Input: part model. Units: mm. Frame: model coordinates. A direction names the side the tool comes from. Round coordinates to 2 decimals unless told otherwise and drop trailing zeros. Order: outer loops, then holes, each group sorted by start corner. A loop starts at its lowest first (then second) coordinate and runs counter-clockwise, first axis right, second up. Notation, with made-up numbers: M -18.75,63.25 L 30.25,63.25 A28 ccw 30.25,85.25 Z; hole C 83,-18.75 d3. An arc over 180 degrees is marked long. One line per question, with ' | ' between items.
```python
from build123d import *

# Parameters (mm, degrees)
BOSS_EXTRUDE1_DEPTH = 20
SKETCH2_W           = 1
SKETCH2_H           = 2.5
SKETCH2_H_2         = 10
BOSS_EXTRUDE2_DEPTH = 2.5
SKETCH2_3_R         = 2.5
CUT_EXTRUDE1_DEPTH  = 35.641016151
SKETCH3_W           = 1
SKETCH3_H           = 10
BOSS_EXTRUDE3_DEPTH = 2.5
SKETCH4_W           = 1
SKETCH4_H           = 10
SKETCH4_W_2         = 10
SKETCH4_H_2         = 1
BOSS_EXTRUDE4_DEPTH = 2.5
SKETCH4_3_R         = 2.5
CUT_EXTRUDE2_DEPTH  = 37.142080737
SKETCH5_R           = 6
CUT_EXTRUDE3_DEPTH  = 17
SKETCH6_R           = 6
CUT_EXTRUDE4_DEPTH  = 17
SKETCH7_R           = 6
CUT_EXTRUDE5_DEPTH  = 17


with BuildPart() as part:
    # Sketch1 → Boss-Extrude1 (new body)
    with BuildSketch(Plane(origin=(0, 0, 0), x_dir=(1, 0, 0), z_dir=(0, 1, 0))):
        Polygon((0, 7.5), (3, 7.5), (3, 12.5), (0, 12.5), (0, 20), (20, 20), (20, 0), (0, 0), align=None)
    extrude(amount=BOSS_EXTRUDE1_DEPTH)

    # Sketch2 → Boss-Extrude2 (add)
    with BuildSketch(Plane(origin=(0, 20, 0), x_dir=(1, 0, 0), z_dir=(0, 1, 0))):
        with Locations((2.5, 6.25)):
            Rectangle(SKETCH2_W, SKETCH2_H)
        with Locations((2.5, 13.75)):
            Rectangle(SKETCH2_W, SKETCH2_H)
        with Locations((17.5, 10)):
            Rectangle(SKETCH2_W, SKETCH2_H_2)
    extrude(amount=BOSS_EXTRUDE2_DEPTH)

    # Sketch2_3 → Cut-Extrude1 (cut, through all)
    with BuildSketch(Plane(origin=(0, 20, 0), x_dir=(1, 0, 0), z_dir=(0, 1, 0))):
        with Locations(Location((10, 10, 0), (0, 0, 270))):
            Circle(SKETCH2_3_R)
    extrude(amount=-CUT_EXTRUDE1_DEPTH, mode=Mode.SUBTRACT)

    # Sketch3 → Boss-Extrude3 (add)
    with BuildSketch(Plane.ZY):
        with Locations((-2.5, 10)):
            Rectangle(SKETCH3_W, SKETCH3_H)
        with Locations((-17.5, 10)):
            Rectangle(SKETCH3_W, SKETCH3_H)
    extrude(amount=BOSS_EXTRUDE3_DEPTH)

    # Sketch4 → Boss-Extrude4 (add)
    with BuildSketch(Plane(origin=(0, 0, -20), x_dir=(-1, 0, 0), z_dir=(0, 0, -1))):
        with Locations((-17.5, 10)):
            Rectangle(SKETCH4_W, SKETCH4_H)
        with Locations((-2.5, 10)):
            Rectangle(SKETCH4_W, SKETCH4_H)
        with Locations((-10, 2.5)):
            Rectangle(SKETCH4_W_2, SKETCH4_H_2)
    extrude(amount=BOSS_EXTRUDE4_DEPTH)

    # Sketch4_3 → Cut-Extrude2 (cut, through all)
    with BuildSketch(Plane(origin=(0, 0, -20), x_dir=(-1, 0, 0), z_dir=(0, 0, -1))):
        with Locations((-10, 10)):
            Circle(SKETCH4_3_R)
    extrude(amount=-CUT_EXTRUDE2_DEPTH, mode=Mode.SUBTRACT)

    # Sketch5 → Cut-Extrude3 (cut)
    with BuildSketch(Plane(origin=(20, 0, 0), x_dir=(0, 0, -1), z_dir=(1, 0, 0))):
        with Locations((10, 10)):
            Circle(SKETCH5_R)
    extrude(amount=-CUT_EXTRUDE3_DEPTH, mode=Mode.SUBTRACT)

    # Sketch6 → Cut-Extrude4 (cut)
    with BuildSketch(Plane.XY):
        with Locations((10, 10)):
            Circle(SKETCH6_R)
    extrude(amount=-CUT_EXTRUDE4_DEPTH, mode=Mode.SUBTRACT)

    # Sketch7 → Cut-Extrude5 (cut)
    with BuildSketch(Plane.XZ):
        with Locations(Location((10, -10, 0), (0, 0, 270))):
            Circle(SKETCH7_R)
    extrude(amount=-CUT_EXTRUDE5_DEPTH, mode=Mode.SUBTRACT)


solid = part.part
```
Item 1: Section query B-B, the plane z = -21. Return loops of the section in (x, y), plus the area to 3 significant figures.
Report:
outline: M 2,5 L 3,5 L 3,15 L 2,15 Z; M 5,2 L 15,2 L 15,3 L 5,3 Z; M 17,5 L 18,5 L 18,15 L 17,15 Z | area: 30.0 mm²
Item 2: Section query D-D, the plane y = 10. Give the number of separate pieces and of enclosed holes in the cut face, plus the area to 3 significant figures.
Report:
separate pieces: 4 | enclosed holes: 0 | area: 116 mm²
Item 3: Section query A-A, the plane x = 10. Return loops of the section in (y, z).
Report:
outline: M 0,-20 L 2,-20 L 2,-22.5 L 3,-22.5 L 3,-20 L 7.5,-20 L 7.5,-17 L 4,-17 L 4,-16 L 0,-16 Z; M 0,-4 L 4,-4 L 4,0 L 0,0 Z; M 12.5,-20 L 20,-20 L 20,-12.5 L 17,-12.5 L 17,-16 L 16,-16 L 16,-17 L 12.5,-17 Z; M 16,-4 L 17,-4 L 17,-7.5 L 20,-7.5 L 20,0 L 16,0 Z
Item 4: Access query for faces 1 (the flat face through (3, 18, -10)), 2 (the flat face through (10, 2, -21)), 3 (the flat face through (17, 10, -21)), 4 (the cylindrical face through (14.06, 2.2, -5.58)), 5 (the flat face through (2, 10, -21)). Directions: +Z, -Z, +X, -X, +Y, -Y. A direction counts if a zero-diameter tool reaches every point of the face in a straight line with its end or side. Return the directions, or none.
Report:
face 1: -X, +Y, -Y | face 2: -Z, +X, -X, -Y | face 3: -Z, +Y, -Y | face 4: -Y | face 5: -Z, -X, +Y, -Y
Item 5: Line query: line 1 along Z through (x, y) = (3.9, 10); line 2 along Z through (x, y) = (14.25, 4.25); line 3 along X through (y, z) = (11.5, -13). Output: solid intervals per line, ascending. Write a range as from..to.
Report:
line 1: -20..-16, -4..0 | line 2: -20..-14.24, -5.76..0 | line 3: 0..3
Item 6: Mould query, pull axis Y, two halves, no side actions, for faces 6 (the cylindrical face through (17.8, 14.06, -5.58)), 7 (the flat face through (-1, 10, -3)), 8 (the flat face through (2.5, 22.5, -13.8)), 9 (the flat face through (3, 10, -6)). Classes: +Y half, -Y half, draft (parallel to the pull), parting line (faces both ways), or undercut.
Report:
face 6: undercut | face 7: draft | face 8: +Y half | face 9: undercut
Item 7: Section query C-C, the plane z = -10. Return loops of the section in (x, y), plus the area to 3 significant figures.
Report:
outline: M 3,0 L 4,0 L 4,4 L 3,4 Z; M 3,16 L 4,16 L 4,17 L 7.5,17 L 7.5,20 L 3,20 Z; M 12.5,17 L 16,17 L 16,16 L 20,16 L 20,20 L 18,20 L 18,22.5 L 17,22.5 L 17,20 L 12.5,20 Z; M 16,0 L 20,0 L 20,4 L 16,4 Z | area: 63.5 mm²
Item 8: First-contact query: pin 1 (5 mm diameter, centred on x = 8, y = 3.5, fed in from -Z); pin 2 (9.5 mm diameter, centred on x = 10, y = 10, fed in from +Z); pin 3 (1.1 mm diameter, centred on y = 7.5, z = -14, fed in from +X); pin 4 (3 mm diameter, centred on y = 22, z = -8, fed in from +X). Flat tips, straight axial feed; report the tip coordinate or a pass-through.
Report:
pin 1: z = -22.5 | pin 2: z = -17 | pin 3: x = 3 | pin 4: x = 18
